from build123d import *

# Parameters (mm, degrees)
F0_W     = 600
F0_H     = 150
F0_W_2   = 8
F0_H_2   = 133.593111
F1_DEPTH = 5
F2_W     = 600
F2_H     = 150
F3_DEPTH = 1


with BuildPart() as f1:
    # F0 (on Top) → F1 (new body)
    with BuildSketch(Plane.XY):
        with Locations((11.197913, -45.502181)):
            Rectangle(F0_W, F0_H)
        with Locations((-276.802087, -46.449782)):
            Rectangle(F0_W_2, F0_H_2, mode=Mode.SUBTRACT)
        with Locations((-260.802087, -46.449782)):
            Rectangle(F0_W_2, F0_H_2, mode=Mode.SUBTRACT)
        with Locations((-244.802087, -46.449782)):
            Rectangle(F0_W_2, F0_H_2, mode=Mode.SUBTRACT)
        with Locations((-228.802087, -46.449782)):
            Rectangle(F0_W_2, F0_H_2, mode=Mode.SUBTRACT)
        with Locations((-212.802087, -46.449782)):
            Rectangle(F0_W_2, F0_H_2, mode=Mode.SUBTRACT)
        with Locations((-196.802087, -46.449782)):
            Rectangle(F0_W_2, F0_H_2, mode=Mode.SUBTRACT)
        with Locations((-180.802087, -46.449782)):
            Rectangle(F0_W_2, F0_H_2, mode=Mode.SUBTRACT)
        with Locations((-164.802087, -46.449782)):
            Rectangle(F0_W_2, F0_H_2, mode=Mode.SUBTRACT)
        with Locations((-148.802087, -46.449782)):
            Rectangle(F0_W_2, F0_H_2, mode=Mode.SUBTRACT)
        with Locations((-132.802087, -46.449782)):
            Rectangle(F0_W_2, F0_H_2, mode=Mode.SUBTRACT)
        with Locations((-116.802087, -46.449782)):
            Rectangle(F0_W_2, F0_H_2, mode=Mode.SUBTRACT)
        with Locations((-100.802087, -46.449782)):
            Rectangle(F0_W_2, F0_H_2, mode=Mode.SUBTRACT)
        with Locations((-84.802087, -46.449782)):
            Rectangle(F0_W_2, F0_H_2, mode=Mode.SUBTRACT)
        with Locations((-68.802087, -46.449782)):
            Rectangle(F0_W_2, F0_H_2, mode=Mode.SUBTRACT)
        with Locations((-52.802087, -46.449782)):
            Rectangle(F0_W_2, F0_H_2, mode=Mode.SUBTRACT)
        with Locations((-36.802087, -46.449782)):
            Rectangle(F0_W_2, F0_H_2, mode=Mode.SUBTRACT)
        with Locations((-20.802087, -46.449782)):
            Rectangle(F0_W_2, F0_H_2, mode=Mode.SUBTRACT)
        with Locations((-4.802087, -46.449782)):
            Rectangle(F0_W_2, F0_H_2, mode=Mode.SUBTRACT)
        with Locations((11.197913, -46.449782)):
            Rectangle(F0_W_2, F0_H_2, mode=Mode.SUBTRACT)
        with Locations((27.197913, -46.449782)):
            Rectangle(F0_W_2, F0_H_2, mode=Mode.SUBTRACT)
        with Locations((43.197913, -46.449782)):
            Rectangle(F0_W_2, F0_H_2, mode=Mode.SUBTRACT)
        with Locations((59.197913, -46.449782)):
            Rectangle(F0_W_2, F0_H_2, mode=Mode.SUBTRACT)
        with Locations((75.197913, -46.449782)):
            Rectangle(F0_W_2, F0_H_2, mode=Mode.SUBTRACT)
        with Locations((91.197913, -46.449782)):
            Rectangle(F0_W_2, F0_H_2, mode=Mode.SUBTRACT)
        with Locations((107.197913, -46.449782)):
            Rectangle(F0_W_2, F0_H_2, mode=Mode.SUBTRACT)
        with Locations((123.197913, -46.449782)):
            Rectangle(F0_W_2, F0_H_2, mode=Mode.SUBTRACT)
        with Locations((139.197913, -46.449782)):
            Rectangle(F0_W_2, F0_H_2, mode=Mode.SUBTRACT)
        with Locations((155.197913, -46.449782)):
            Rectangle(F0_W_2, F0_H_2, mode=Mode.SUBTRACT)
        with Locations((171.197913, -46.449782)):
            Rectangle(F0_W_2, F0_H_2, mode=Mode.SUBTRACT)
        with Locations((187.197913, -46.449782)):
            Rectangle(F0_W_2, F0_H_2, mode=Mode.SUBTRACT)
        with Locations((203.197913, -46.449782)):
            Rectangle(F0_W_2, F0_H_2, mode=Mode.SUBTRACT)
        with Locations((219.197913, -46.449782)):
            Rectangle(F0_W_2, F0_H_2, mode=Mode.SUBTRACT)
        with Locations((235.197913, -46.449782)):
            Rectangle(F0_W_2, F0_H_2, mode=Mode.SUBTRACT)
        with Locations((251.197913, -46.449782)):
            Rectangle(F0_W_2, F0_H_2, mode=Mode.SUBTRACT)
        with Locations((267.197913, -46.449782)):
            Rectangle(F0_W_2, F0_H_2, mode=Mode.SUBTRACT)
        with Locations((283.197913, -46.449782)):
            Rectangle(F0_W_2, F0_H_2, mode=Mode.SUBTRACT)
        with Locations((299.197913, -46.449782)):
            Rectangle(F0_W_2, F0_H_2, mode=Mode.SUBTRACT)
    extrude(amount=F1_DEPTH)

    # F2 (on face) → F3 (join)
    with BuildSketch(Plane(origin=(0, 0, 0), x_dir=(1, 0, 0), z_dir=(0, 0, -1))):
        with Locations((11.197913, 45.502181)):
            Rectangle(F2_W, F2_H)
    extrude(amount=F3_DEPTH)


solid = f1.part
Input: part model. Units: mm. Frame: model coordinates. Coordinates: 2 decimals unless noted, no trailing zeros. Write each question's results on one line, items separated by ' | '. Start each with the question number.
Q1. Ray query, line 1 (Y direction, x = -3.5, z = 1.7); line 2 (Z direction, x = 154, y = -76). Return the intervals inside material, ascending. Write a range as from..to.
Q2. Section A-A, the plane z = 2. State how many separate pieces and enclosed holes the cut face has, plus the area to 3 significant figures.
Q3. Pin query (flat end, axial travel): pin 1 (4 mm diameter, centred on x = -243.5, y = -70, fed in from +Z). Return the tip coordinate at first contact, or that it passes through.
Found:
1) line 1: -120.5..-113.25, 20.35..29.5 | line 2: -1..0
2) separate pieces: 1 | enclosed holes: 37 | area: 50,500 mm2
3) pin 1: z = 0
